Could you check a few things on this model? Use its own coordinates, in mm. Face numbers are marked on the shaded views. A direction names the side the tool comes from. Give positions to 0.01 mm unless a question says otherwise; leave off trailing zeros. Loops run counter-clockwise (first coordinate to the right, second up) from the corner with the lowest first, then second, coordinate; pieces in that order, holes last. Notation, with made-up numbers: (73, 17.5) - (126, 17.5) arc R11 cw to (126, 31.5) - close; hole circle Ø11 at (70.25, 62.25). An arc over 180 degrees is marked (long way). Write each question's results on one line, items separated by ' | '. Start each with the question number.
1) I want a section at A-A, the plane x = 125. Write out the boundary of the cut face in (y, z).
2) I'm going to push flat-ended pins straight in: pin 1 (1.5 mm diameter, centred on x = 81, y = 2.5, fed in from +Z); pin 2 (1.5 mm diameter, centred on x = -105, y = 3, fed in from -Z); pin 3 (12 mm diameter, centred on x = 92, y = -9, fed in from -Z); pin 4 (5 mm diameter, centred on x = 125, z = 0, fed in from -Y). Where does each tip first touch, or does it pass through?
3) I want a section at B-B, the plane x = 63. Write out the boundary of the cut face in (y, z).
4) If I drill on probe 1 along X at (y, z) = (-4, 0); probe 2 along X at (y, z) = (-9.5, 0); probe 3 along X at (y, z) = (11.5, -4), over which ranges is the centre line in solid material (lowest first)? Write a range as [from, to].
5) On a 3-axis mill with a long thin cutter (end or side, diameter ignored), from which of +Z, -Z, +X, -X, +Y, -Y can I reach the whole of each face in a straight line? I mean the marked faces 1 and 2. Say none if no direction works.
Solid Edge part; units mm, degrees
sketch "Sketch1" plane through (0, 0, 0) normal (1, 0, 0) x (0, 1, 0)
  circle A0 centre (0, 0) radius 10
extrude "Protrusion1" add sketch "Sketch1" along normal mid plane 210
sketch "Sketch2" plane through (-105, 0, 0) normal (-1, 0, 0) x (0, -1, 0)
  circle A0 centre (0, 0) radius 6
extrude "ExtrudedProtrusion_2" add sketch "Sketch2" along normal blind 18
sketch "Sketch3" plane through (-123, 0, 0) normal (-1, 0, 0) x (0, -1, 0)
  circle A0 centre (0, 0) radius 5
extrude "ExtrudedProtrusion_3" add sketch "Sketch3" along normal blind 22
sketch "Sketch4" plane through (105, 0, 0) normal (1, 0, 0) x (0, 1, 0)
  circle A0 centre (0, 0) radius 16
extrude "ExtrudedProtrusion_4" add sketch "Sketch4" along normal blind 40
cosmetic_thread "Thread1"
cosmetic_thread "Thread_2" thread depth 170
fillet "Round_1" radius 3 2 edges at (145, -16, 0) (105, -16, 0)
sketch "Sketch5" plane through (0, 0, 0) normal (0, -1, 0) x (1, 0, 0)
  circle A0 centre (125, 0) radius 3
extrude "ExtrudedCutout_2" cut sketch "Sketch5" along normal mid plane 57.4711
sketch "Sketch6" plane through (0, 0, 0) normal (0, 0, 1) x (1, 0, 0)
  circle A0 centre (125, 0) radius 3
extrude "ExtrudedCutout_3" cut sketch "Sketch6" along normal mid plane 101.3588
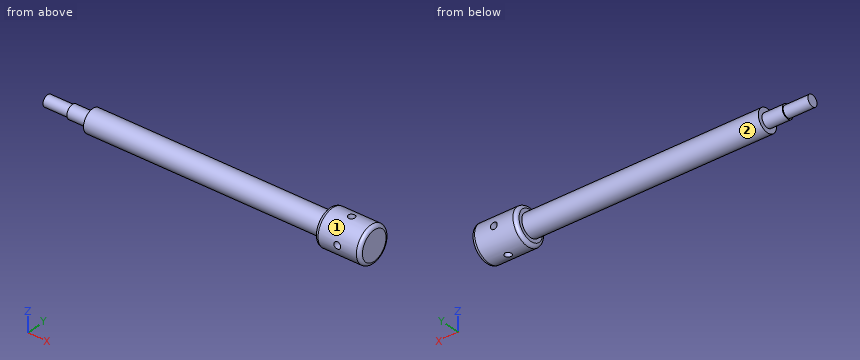
Answers:
1) outline: (-15.72, -3) arc R16 ccw to (-3, -15.72) - (-3, -3) - close; (-15.72, 3) - (-3, 3) - (-3, 15.72) arc R16 ccw to start; (3, -15.72) arc R16 ccw to (15.72, -3) - (3, -3) - close; (3, 3) - (15.72, 3) arc R16 ccw to (3, 15.72) - close
2) pin 1: stops at z = 9.85 | pin 2: stops at z = -9.74 | pin 3: stops at z = -9.54 | pin 4: passes through
3) outline: circle Ø20 at (0, 0)
4) probe 1: x = [-145, 122], [128, 145] | probe 2: x = [-105, 122], [128, 145] | probe 3: x = [105, 145]
5) face 1: +X, -X | face 2: -X
